Source: CAD feature listing. Evaluate the final solid. Frame: model axes, mm. A direction names the side the tool comes from. Give positions to 0.01 mm unless a question says otherwise; leave off trailing zeros. Write each loop counter-clockwise with the first axis right and the second up, starting at its lowest first coordinate (ties: lowest second). Pieces come first, ordered by that corner, then holes. Notation, with made-up numbers: (22, -22) - (33, -22) arc R19 ccw to (33, -12) - close; hole circle Ø3 at (62, -32). An arc over 180 degrees is marked (long way). One line per question, with ' | ' between items. Start each with the question number.
(1) Draft query along X for faces 1 (the flat face through (10, 0, 4.762)), 2 (the flat face through (10, 0, -0.794)). Return one class per face: +X half, -X half, draft (parallel to the pull), parting line (faces both ways), or undercut.
(2) Section D-D, the plane x = 12.7. Return loops of the section in (y, z).
(3) Section A-A, the plane x = 8.5. Return loops of the section in (y, z).
(4) Access query for faces 3 (the flat face through (10, 0, 0)), 4 (the flat face through (10, 0, 5.556)), 5 (the flat face through (6, 0, -0.54)), 6 (the flat face through (13, 0, 5.302)). Directions: +Z, -Z, +X, -X, +Y, -Y. A direction counts if a zero-diameter tool reaches every point of the face in a straight line with its end or side. Return the directions, or none.
(5) Ray query, line 1 (Y direction, x = 6.35, z = 5.4); line 2 (Z direction, x = 7, y = -1.4); line 3 (X direction, y = -0.65, z = 3.5). Return the intervals inside material, ascending. Write a range as [from, to].
(6) Section B-B, the plane y = 1.45. Return loops of the section in (x, z).
(7) Pin query (flat end, axial travel): pin 1 (3 mm diameter, centred on y = 2, z = 0, fed in from -X); pin 2 (0.5 mm diameter, centred on x = 12.5, y = 0, fed in from +Z); pin 3 (1 mm diameter, centred on x = 6.35, y = 0, fed in from -Z); pin 4 (1.7 mm diameter, centred on x = 6.5, y = 0, fed in from -Z). Return the tip coordinate at first contact, or that it passes through.
```python
from build123d import *

# Parameters (mm, degrees)
SKETCH2_R           = 2.38125
SKETCH2_R_2         = 1.190625
BOSS_EXTRUDE1_DEPTH = 0.79375
SKETCH3_R           = 2.69875
SKETCH3_R_2         = 1.190625
BOSS_EXTRUDE2_DEPTH = 0.79375
BOSS_EXTRUDE3_START = 0.79375
SKETCH3_4_R         = 1.190625
BOSS_EXTRUDE3_DEPTH = 3.175
SKETCH4_R           = 0.79375
CUT_EXTRUDE1_DEPTH  = 0.254


with BuildPart() as part:
    # Sketch2 → Boss-Extrude1 (new body)
    # profile 1 of 3: a face of its own
    with BuildSketch(Plane.XY):
        Circle(SKETCH2_R)
        Circle(SKETCH2_R_2, mode=Mode.SUBTRACT)
    # profile 2 of 3: a face of its own
    with BuildSketch(Plane.XY):
        with BuildLine():
            ThreePointArc((1.5875, 1.774878957), (2.1737739, 0.972141242), (2.38125, 0))
            ThreePointArc((2.38125, 0), (2.1737739, -0.972141242), (1.5875, -1.774878957))
            ThreePointArc((1.5875, -1.774878957), (3.175, -1.168507914), (4.7625, -1.774878957))
            ThreePointArc((4.7625, -1.774878957), (3.96875, 0), (4.7625, 1.774878957))
            ThreePointArc((4.7625, 1.774878957), (3.175, 1.168507914), (1.5875, 1.774878957))
        make_face()
    # profile 3 of 3: a face of its own
    with BuildSketch(Plane.XY):
        with Locations((6.35, 0)):
            Circle(SKETCH2_R)
        with Locations((6.35, 0)):
            Circle(SKETCH2_R_2, mode=Mode.SUBTRACT)
    extrude(amount=BOSS_EXTRUDE1_DEPTH)


with BuildPart() as body_2:
    # Sketch3 → Boss-Extrude2 (new body)
    # profile 1 of 4: a face of its own
    with BuildSketch(Plane(origin=(0, 0, 0), x_dir=(-1, 0, 0), z_dir=(0, 0, -1))):
        with Locations((-12.7, 0)):
            Circle(SKETCH3_R)
        with Locations((-12.7, 0)):
            Circle(SKETCH3_R_2, mode=Mode.SUBTRACT)
    # profile 2 of 4: a face of its own
    with BuildSketch(Plane(origin=(0, 0, 0), x_dir=(-1, 0, 0), z_dir=(0, 0, -1))):
        with BuildLine():
            ThreePointArc((-3.65125, 0), (-3.737895814, 0.678353361), (-3.99226957, 1.313148424))
            ThreePointArc((-3.99226957, 1.313148424), (-4.399347966, 1.507376065), (-4.7625, 1.774878957))
            ThreePointArc((-4.7625, 1.774878957), (-8.73125, 0), (-4.7625, -1.774878957))
            ThreePointArc((-4.7625, -1.774878957), (-4.399347966, -1.507376065), (-3.99226957, -1.313148424))
            ThreePointArc((-3.99226957, -1.313148424), (-3.737895814, -0.678353361), (-3.65125, 0))
        make_face()
        with Locations(Location((-6.35, 0, 0), (0, 0, 180))):
            Circle(SKETCH3_R_2, mode=Mode.SUBTRACT)
    # profile 3 of 4: a face of its own
    with BuildSketch(Plane(origin=(0, 0, 0), x_dir=(-1, 0, 0), z_dir=(0, 0, -1))):
        with BuildLine():
            ThreePointArc((-3.99226957, 1.313148424), (-5.769279961, 2.63552951), (-7.9375, 2.182451675))
            ThreePointArc((-7.9375, 2.182451675), (-9.04875, 0), (-7.9375, -2.182451675))
            ThreePointArc((-7.9375, -2.182451675), (-5.769279961, -2.63552951), (-3.99226957, -1.313148424))
            ThreePointArc((-3.99226957, -1.313148424), (-4.399347966, -1.507376065), (-4.7625, -1.774878957))
            ThreePointArc((-4.7625, -1.774878957), (-8.73125, 0), (-4.7625, 1.774878957))
            ThreePointArc((-4.7625, 1.774878957), (-4.399347966, 1.507376065), (-3.99226957, 1.313148424))
        make_face()
    # profile 4 of 4: a face of its own
    with BuildSketch(Plane(origin=(0, 0, 0), x_dir=(-1, 0, 0), z_dir=(0, 0, -1))):
        with BuildLine():
            ThreePointArc((-7.9375, -2.182451675), (-9.04875, 0), (-7.9375, 2.182451675))
            ThreePointArc((-7.9375, 2.182451675), (-9.525, 1.666153349), (-11.1125, 2.182451675))
            ThreePointArc((-11.1125, 2.182451675), (-10.295055387, 1.224537859), (-10.00125, 0))
            ThreePointArc((-10.00125, 0), (-10.295055387, -1.224537859), (-11.1125, -2.182451675))
            ThreePointArc((-11.1125, -2.182451675), (-9.525, -1.666153349), (-7.9375, -2.182451675))
        make_face()
    extrude(amount=BOSS_EXTRUDE2_DEPTH)

    # Sketch3<4> → Boss-Extrude3 (add)
    with BuildSketch(Plane(origin=(0, 0, 0), x_dir=(-1, 0, 0), z_dir=(0, 0, -1)).offset(BOSS_EXTRUDE3_START)):
        with Locations(Location((-6.35, 0, 0), (0, 0, 180))):
            Circle(SKETCH3_4_R)
        with Locations((-12.7, 0)):
            Circle(SKETCH3_4_R)
    extrude(amount=-BOSS_EXTRUDE3_DEPTH)


with BuildPart() as body_3:
    # Mirror1: mirrored copy
    add(body_2.part.mirror(Plane(origin=(6.35, 0, 2.38125), x_dir=(1, 0, 0), z_dir=(0, 0, -1))))


with BuildPart() as body_4:
    # Mirror1 2: mirrored copy
    add(part.part.mirror(Plane(origin=(6.35, 0, 2.38125), x_dir=(1, 0, 0), z_dir=(0, 0, -1))))


with BuildPart() as body_2_1:
    add(body_2.part)

    # Combine1: union body 3
    add(body_3.part)

    # Sketch4 → Cut-Extrude1 (cut)
    with BuildSketch(Plane(origin=(0, 0, -0.79375), x_dir=(-1, 0, 0), z_dir=(0, 0, -1))):
        with Locations((-6.35, 0)):
            Circle(SKETCH4_R)
        with Locations((-12.7, 0)):
            Circle(SKETCH4_R)
    cut_extrude1 = extrude(amount=-CUT_EXTRUDE1_DEPTH, mode=Mode.SUBTRACT)

    # Mirror2: Cut-Extrude1 across plane
    add(cut_extrude1.mirror(Plane.XY.offset(2.38125)), mode=Mode.SUBTRACT)


solid = body_2_1.part
```
Check sheet entries:
1) face 1: undercut | face 2: draft
2) outline: (-2.7, -0.79) - (-0.79, -0.79) - (-0.79, -0.54) - (0.79, -0.54) - (0.79, -0.79) - (2.7, -0.79) - (2.7, 0) - (1.19, 0) - (1.19, 4.76) - (2.7, 4.76) - (2.7, 5.56) - (0.79, 5.56) - (0.79, 5.3) - (-0.79, 5.3) - (-0.79, 5.56) - (-2.7, 5.56) - (-2.7, 4.76) - (-1.19, 4.76) - (-1.19, 0) - (-2.7, 0) - close
3) outline: (-1.87, -0.79) - (1.87, -0.79) - (1.87, 0) - (-1.87, 0) - close; (-1.87, 4.76) - (1.87, 4.76) - (1.87, 5.56) - (-1.87, 5.56) - close
4) face 3: none | face 4: +Z, +X, -X, +Y, -Y | face 5: -Z | face 6: +Z
5) line 1: [-2.7, -0.79], [0.79, 2.7] | line 2: [-0.79, 0], [4.76, 5.56] | line 3: [5.35, 7.35], [11.7, 13.7]
6) outline: (4.07, -0.79) - (14.98, -0.79) - (14.98, 0) - (4.07, 0) - close; (4.07, 4.76) - (14.98, 4.76) - (14.98, 5.56) - (4.07, 5.56) - close
7) pin 1: x = 3.7 | pin 2: z = 5.3 | pin 3: z = -0.54 | pin 4: z = -0.79
